Read the model definition and answer for the solid it produces. Units are mm, in the model's axes. A direction names the side the tool comes from. Give positions to 0.01 mm unless a question says otherwise; leave off trailing zeros. Loops run counter-clockwise (first coordinate to the right, second up) from the corner with the lowest first, then second, coordinate; pieces in that order, holes last.
(1) Find section D-D, the plane x = 15.5. Write down the section's boundary in (y, z).
(2) Determine the mould class of faces 1 (the face through (28.2, 86.3, 11.9)), 2 (the face through (20, 87.1, 12)), 3 (the face through (0.805, 42.045, 14.007)), 4 (the face through (1, 0, 12)) for opening direction Y: pulls with the +Y half, pulls with the -Y half, needs draft (parallel to the pull), parting line crosses it, or undercut.
(3) Find section C-C, the plane z = 12.5. Write down the section's boundary in (x, y), then the cut area to 3 significant figures.
(4) Straight lines are drawn through the part: probe 1 along Y at (x, z) = (1.1, 10); probe 2 along Z at (x, y) = (10, 86); probe 3 along X at (y, z) = (79.5, 6.75). For each, find the intervals that lie inside material, in ascending order.
(5) Find section A-A, the plane x = 10. Write down the section's boundary in (y, z).
(6) Each of these flat-tipped pins is pushed along its axis until it touches: P1, Ø1.2, axis at y = 28.2, z = 15, coming from the +X side; P2, Ø8, axis at y = 44.5, z = 16.5, coming from the -X side; P3, Ø8, axis at x = 19, z = 11.5, coming from the -Y side; P4, Ø2.5, axis at y = 10, z = 15, coming from the +X side. Where does it stop, or does it pass through?
(7) Which of the six approach directions +Z, -Z, +X, -X, +Y, -Y give full straight-line access (tool end or side, diameter ignored) to faces 5 (the face through (0.8, 10.31, 14.02)), 6 (the face through (21, 85.512, 12))?
(8) Find section B-B, the plane y = 43.2. Write down the section's boundary in (x, z), then the cut area to 3 significant figures.
```python
from build123d import *

# Parameters (mm, degrees)
BOSS_EXTRUDE1_DEPTH   = 25
F_6_CLEARANCE_HOLE1_D = 3.7973
F_1_CLEARANCE_HOLE2_D = 2.0574
F_6_CLEARANCE_HOLE2_D = 3.7973


with BuildPart() as part:
    # Sketch2 → Boss-Extrude1 (new body)
    with BuildSketch(Plane.XY):
        Polygon((0, 0), (0, 87.1), (40, 87.1), (40, 85.5125), (1.5875, 85.5125), (1.5875, 0), align=None)
    extrude(amount=BOSS_EXTRUDE1_DEPTH)

    # #6 Clearance Hole1 (through all)
    with Locations(Plane(origin=(0, 87.1, 0), x_dir=(1, 0, 0), z_dir=(0, 1, 0))):
        with Locations((10, -12.5), (30, -12.5)):
            Hole(F_6_CLEARANCE_HOLE1_D / 2)

    # #1 Clearance Hole2 (through all)
    with Locations(Plane.ZY):
        with Locations((15, 10), (15, 28.2), (10, 10), (10, 28.2)):
            Hole(F_1_CLEARANCE_HOLE2_D / 2)

    # #6 Clearance Hole2 (through all)
    with Locations(Plane.ZY):
        with Locations((12.5, 43.2)):
            Hole(F_6_CLEARANCE_HOLE2_D / 2)


solid = part.part
```
Entries:
1. outline: (85.51, 0) - (87.1, 0) - (87.1, 25) - (85.51, 25) - close
2. face 1: needs draft
2. face 2: pulls with the +Y half
2. face 3: undercut
2. face 4: pulls with the -Y half
3. outline: (0, 0) - (1.59, 0) - (1.59, 41.3) - (0, 41.3) - close; (0, 45.1) - (1.59, 45.1) - (1.59, 85.51) - (8.1, 85.51) - (8.1, 87.1) - (0, 87.1) - close; (11.9, 85.51) - (28.1, 85.51) - (28.1, 87.1) - (11.9, 87.1) - close; (31.9, 85.51) - (40, 85.51) - (40, 87.1) - (31.9, 87.1) - close
3. area: 181 mm2
4. probe 1: y = 0 to 8.97, 11.03 to 27.17, 29.23 to 87.1
4. probe 2: z = 0 to 10.6, 14.4 to 25
4. probe 3: x = 0 to 1.59
5. outline: (85.51, 0) - (87.1, 0) - (87.1, 10.6) - (85.51, 10.6) - close; (85.51, 14.4) - (87.1, 14.4) - (87.1, 25) - (85.51, 25) - close
6. P1: passes through
6. P2: stops at x = 0
6. P3: stops at y = 85.51
6. P4: stops at x = 1.59
7. face 5: +X, -X
7. face 6: +Z, -Z, +X, -Y
8. outline: (0, 0) - (1.59, 0) - (1.59, 10.6) - (0, 10.6) - close; (0, 14.4) - (1.59, 14.4) - (1.59, 25) - (0, 25) - close
8. area: 33.7 mm2
